The drawing under review shows one solid part. Ordinate dimensions are in mm from its lowest x, y, z. Coordinates: 2 decimals unless noted, no trailing zeros. Loops run counter-clockwise (first coordinate to the right, second up) from the corner with the lowest first, then second, coordinate; pieces in that order, holes last. Notation, with made-up numbers: M -36,71 L -8,71 A26 ccw -8,97 Z; hole C -34,46 d10. An arc over 180 degrees is marked long. Return JSON: item names as keys, results as strings.
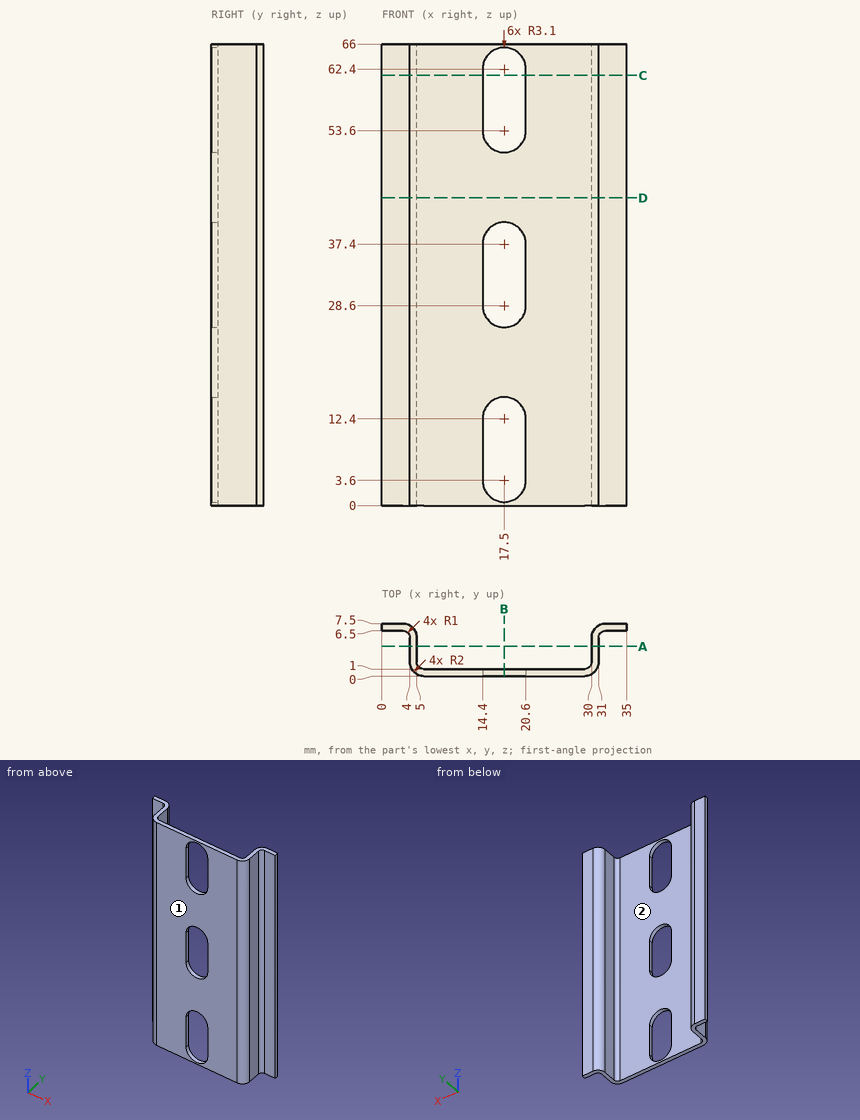
1. Add section C-C on z = 61.5. Give the boundary of the cut face in (x, y), plus the area to 3 significant figures.
Check values:
{"outline": "M 0,6.5 L 3,6.5 A1 cw 4,5.5 L 4,2 A2 ccw 6,0 L 14.4,0 L 14.4,1 L 6,1 A1 cw 5,2 L 5,5.5 A2 ccw 3,7.5 L 0,7.5 Z; M 20.6,0 L 29,0 A2 ccw 31,2 L 31,5.5 A1 cw 32,6.5 L 35,6.5 L 35,7.5 L 32,7.5 A2 ccw 30,5.5 L 30,2 A1 cw 29,1 L 20.6,1 Z", "area": "39.2 mm²"}
2. Add section D-D on z = 44. Give the boundary of the cut face in (x, y).
Check values:
{"outline": "M 0,6.5 L 3,6.5 A1 cw 4,5.5 L 4,2 A2 ccw 6,0 L 29,0 A2 ccw 31,2 L 31,5.5 A1 cw 32,6.5 L 35,6.5 L 35,7.5 L 32,7.5 A2 ccw 30,5.5 L 30,2 A1 cw 29,1 L 6,1 A1 cw 5,2 L 5,5.5 A2 ccw 3,7.5 L 0,7.5 Z"}
3. Add section B-B on x = 17.5. Give the boundary of the cut face in (y, z).
Check values:
{"outline": "M 0,0 L 1,0 L 1,0.5 L 0,0.5 Z; M 0,15.5 L 1,15.5 L 1,25.5 L 0,25.5 Z; M 0,40.5 L 1,40.5 L 1,50.5 L 0,50.5 Z; M 0,65.5 L 1,65.5 L 1,66 L 0,66 Z"}
4. Add section A-A on y = 4.25. Give the boundary of the cut face in (x, z).
Check values:
{"outline": "M 4,0 L 5,0 L 5,66 L 4,66 Z; M 30,0 L 31,0 L 31,66 L 30,66 Z"}
5. To check wall thickness, follow line 1 (X direction, y = 4.5, z = 26.5); line 2 (Y direction, x = 25.5, z = 43.5); line 3 (Y direction, x = 33, z = 42). State the ranges of each line that lie inside material, in increasing order.
Check values:
{"line 1": "4 to 5, 30 to 31", "line 2": "0 to 1", "line 3": "6.5 to 7.5"}
6. Insertion check: pin 1 Ø5 at (x, z) = (29.5, 58.5) entering from -Y; pin 2 Ø2 at (y, z) = (3.5, 48.5) entering from -X; pin 3 Ø3 at (y, z) = (3.5, 37) entering from +X; pin 4 Ø0.5 at (y, z) = (0.5, 6.5) entering from -X. Each pin has a flat end and moves straight along its axis. Give the tip position at first contact, or say it passes through.
Check values:
{"pin 1": "y = 0", "pin 2": "x = 4", "pin 3": "x = 31", "pin 4": "x = 4.44"}
7. The part is to be moulded in two halves that separate along X. For the marked faces 1 and 2, say which applies: released by +X, released by -X, zero draft, split by the parting line, or undercut.
Check values:
{"face 1": "zero draft", "face 2": "undercut"}
